Here's how the part is built. I have some questions about the finished solid (model axes, mm). A direction names the side the tool comes from. Round coordinates to 2 decimals unless told otherwise and drop trailing zeros. Order: outer loops, then holes, each group sorted by start corner. A loop starts at its lowest first (then second) coordinate and runs counter-clockwise, first axis right, second up. Notation, with made-up numbers: (-24, 11.25) - (1, 11.25) arc R23 ccw to (1, 19.25) - close; hole circle Ø1 at (69.5, 74.5). An arc over 180 degrees is marked (long way). One line per item, written item: value.
from build123d import *

# Parameters (mm, degrees)
BOSS_EXTRUDE1_DEPTH = 5
BOSS_EXTRUDE2_DEPTH = 32
CUT_EXTRUDE2_DEPTH  = 5
CUT_EXTRUDE3_DEPTH  = 5
SKETCH7_R           = 6.75
SKETCH7_R_2         = 1.75
C_L_NG_C_DEPTH      = 146.27301883
SKETCH8_W           = 40
SKETCH8_H           = 10
BOSS_EXTRUDE3_DEPTH = 55
CUT_EXTRUDE5_DEPTH  = 179.966477308
SKETCH10_R          = 1.75
SKETCH10_R_2        = 2.25
C_L_DEPTH           = 121.768719069
BOSS_EXTRUDE4_REACH = 179.37
CUT_EXTRUDE7_DEPTH  = 5
SKETCH14_R          = 4
CUT_EXTRUDE8_DEPTH  = 2.5
CUT_EXTRUDE9_START  = -2.5
SKETCH15_R          = 4
CUT_EXTRUDE9_DEPTH  = 2.5
SKETCH16_W          = 6
SKETCH16_H          = 10.5
CUT_EXTRUDE10_DEPTH = 5
SKETCH20_W          = 110
SKETCH20_H          = 50.06
CUT_EXTRUDE11_DEPTH = 55
SKETCH22_R          = 2
CUT_EXTRUDE12_DEPTH = 5
CUT_EXTRUDE13_DEPTH = 1.5
CUT_EXTRUDE15_DEPTH = 89
SKETCH26_R          = 1.5
CUT_EXTRUDE16_DEPTH = 5


with BuildPart() as part:
    # Sketch1 → Boss-Extrude1 (new body)
    with BuildSketch(Plane(origin=(0, 0, 0), x_dir=(1, 0, 0), z_dir=(0, 1, 0))):
        Polygon((-25, 75), (-25, 42.5), (-70, 42.5), (-70, -42.5), (-25, -42.5), (-25, -75), (77, -75), (77, 75), align=None)
    extrude(amount=BOSS_EXTRUDE1_DEPTH)

    # Sketch3 → Boss-Extrude2 (add)
    with BuildSketch(Plane(origin=(0, 5, 0), x_dir=(1, 0, 0), z_dir=(0, 1, 0))):
        Polygon((-70, 25), (-65, 25), (-65, 37.5), (-17, 37.5), (-17, 27.5), (-12, 27.5), (-12, 42.5), (-70, 42.5), align=None)
        Polygon((-70, -25), (-70, -42.5), (-12, -42.5), (-12, -27.5), (-17, -27.5), (-17, -37.5), (-65, -37.5), (-65, -25), align=None)
    extrude(amount=BOSS_EXTRUDE2_DEPTH)

    # Sketch5 → Cut-Extrude2 (cut)
    with BuildSketch(Plane.ZY.offset(70)):
        Polygon((-25, 37), (-35, 37), (-35, 27), (-25, 5), align=None)
        Polygon((25, 5), (25, 37), (35, 37), (35, 27), align=None)
    extrude(amount=-CUT_EXTRUDE2_DEPTH, mode=Mode.SUBTRACT)

    # Sketch6 → Cut-Extrude3 (cut)
    with BuildSketch(Plane(origin=(-12, 0, 0), x_dir=(0, 0, -1), z_dir=(1, 0, 0))):
        Polygon((-27.5, 37), (-37.5, 37), (-37.5, 12), (-27.5, 5), align=None)
        Polygon((37.5, 12), (27.5, 5), (27.5, 37), (37.5, 37), align=None)
    extrude(amount=-CUT_EXTRUDE3_DEPTH, mode=Mode.SUBTRACT)

    # Sketch7 → c l_ _ng c (cut, through all)
    with BuildSketch(Plane(origin=(0, 0, -42.5), x_dir=(-1, 0, 0), z_dir=(0, 0, -1))):
        with Locations((49, 21)):
            Circle(SKETCH7_R)
        with Locations((25, 30)):
            Circle(SKETCH7_R_2)
        with Locations((25, 12)):
            Circle(SKETCH7_R_2)
        with Locations((58, 30)):
            Circle(SKETCH7_R_2)
        with Locations((58, 12)):
            Circle(SKETCH7_R_2)
    extrude(amount=-C_L_NG_C_DEPTH, mode=Mode.SUBTRACT)

    # Sketch8 → Boss-Extrude3 (add)
    with BuildSketch(Plane(origin=(0, 5, 0), x_dir=(1, 0, 0), z_dir=(0, 1, 0))):
        with Locations((57, -70)):
            Rectangle(SKETCH8_W, SKETCH8_H)
        with Locations((57, 70)):
            Rectangle(SKETCH8_W, SKETCH8_H)
    extrude(amount=BOSS_EXTRUDE3_DEPTH)

    # Sketch9 → Cut-Extrude5 (cut, through all)
    with BuildSketch(Plane(origin=(0, 0, -75), x_dir=(-1, 0, 0), z_dir=(0, 0, -1))):
        Polygon((-77, 0), (-37, 55.055276819), (-37, 60), (-77, 60), align=None)
    extrude(amount=-CUT_EXTRUDE5_DEPTH, mode=Mode.SUBTRACT)

    # Sketch10 → c L (cut, through all)
    with BuildSketch(Plane(origin=(0, 0, 0), x_dir=(-1, 0, 0), z_dir=(0, -1, 0))):
        with Locations(Location((-29, -12, 0), (0, 0, 90))):
            Circle(SKETCH10_R)
        with Locations(Location((-17, -46, 0), (0, 0, 90))):
            Circle(SKETCH10_R)
        with Locations(Location((-17, 46, 0), (0, 0, 90))):
            Circle(SKETCH10_R)
        with Locations(Location((-29, 12, 0), (0, 0, 90))):
            Circle(SKETCH10_R)
        with Locations(Location((-28, -69.5, 0), (0, 0, 90))):
            Circle(SKETCH10_R_2)
        with Locations(Location((8, -69.5, 0), (0, 0, 90))):
            Circle(SKETCH10_R_2)
        with Locations(Location((8, 69.5, 0), (0, 0, 90))):
            Circle(SKETCH10_R_2)
        with Locations(Location((-28, 69.5, 0), (0, 0, 90))):
            Circle(SKETCH10_R_2)
    extrude(amount=-C_L_DEPTH, mode=Mode.SUBTRACT)

    # Sketch11 → Boss-Extrude4 (add, up to next)
    with BuildSketch(Plane(origin=(0, 0, -75), x_dir=(-1, 0, 0), z_dir=(0, 0, -1)), mode=Mode.PRIVATE) as boss_extrude4_sk1:
        Polygon((-37, 55.055276819), (-37, 50.055276819), (-73.36728736, 0), (-77, 0), align=None)
    boss_extrude4_tool1 = extrude(boss_extrude4_sk1.sketch, amount=-BOSS_EXTRUDE4_REACH, mode=Mode.PRIVATE) - part.part
    add(boss_extrude4_tool1.solids().sort_by_distance((56.106222, 26.297459, -75))[0])

    # Sketch13 → Cut-Extrude7 (cut)
    with BuildSketch(Plane(origin=(50.397154283, 36.615675877, 0), x_dir=(0, 0, -1), z_dir=(0.8090169943749486, 0.5877852522924716, 0))):
        Polygon((-7.731971797, -31.499332186), (-52.405674619, -31.039898345), (-48.866988089, -10.026742728), (-4.277711394, -9.567044368), align=None)
        Polygon((53.010105385, -31.499464427), (49.555844988, -9.567176647), (3.94811969, -10.026742728), (7.33, -31.499464427), align=None)
    extrude(amount=-CUT_EXTRUDE7_DEPTH, mode=Mode.SUBTRACT)

    # Sketch14 → Cut-Extrude8 (cut)
    with BuildSketch(Plane(origin=(0, 0, 37.5), x_dir=(-1, 0, 0), z_dir=(0, 0, -1))):
        with Locations((58, 30)):
            Circle(SKETCH14_R)
        with Locations((25, 30)):
            Circle(SKETCH14_R)
        with Locations((25, 12)):
            Circle(SKETCH14_R)
        with Locations((58, 12)):
            Circle(SKETCH14_R)
        with BuildLine():
            Line((38.8, 26.25), (38.8, 15.75))
            ThreePointArc((38.8, 15.75), (36, 12.95), (33.2, 15.75))
            Line((33.2, 15.75), (33.2, 26.25))
            ThreePointArc((33.2, 26.25), (36, 29.05), (38.8, 26.25))
        make_face()
    extrude(amount=-CUT_EXTRUDE8_DEPTH, mode=Mode.SUBTRACT)

    # Sketch15 → Cut-Extrude9 (cut)
    with BuildSketch(Plane.XY.offset(-37.5).offset(CUT_EXTRUDE9_START)):
        with Locations(Location((-25, 30, 0), (0, 0, 180))):
            Circle(SKETCH15_R)
        with Locations(Location((-25, 12, 0), (0, 0, 180))):
            Circle(SKETCH15_R)
        with Locations(Location((-58, 12, 0), (0, 0, 180))):
            Circle(SKETCH15_R)
        with Locations(Location((-58, 30, 0), (0, 0, 180))):
            Circle(SKETCH15_R)
        with BuildLine():
            Line((-33.2, 26.25), (-33.2, 15.75))
            ThreePointArc((-33.2, 15.75), (-36, 12.95), (-38.8, 15.75))
            Line((-38.8, 15.75), (-38.8, 26.25))
            ThreePointArc((-38.8, 26.25), (-36, 29.05), (-33.2, 26.25))
        make_face()
    extrude(amount=CUT_EXTRUDE9_DEPTH, mode=Mode.SUBTRACT)

    # Sketch16 → Cut-Extrude10 (cut)
    with BuildSketch(Plane(origin=(0, 0, 0), x_dir=(-1, 0, 0), z_dir=(0, -1, 0))):
        with Locations((57, 0)):
            Rectangle(SKETCH16_W, SKETCH16_H)
        with Locations((-64, 0)):
            Rectangle(SKETCH16_W, SKETCH16_H)
    extrude(amount=-CUT_EXTRUDE10_DEPTH, mode=Mode.SUBTRACT)

    # Sketch20 → Cut-Extrude11 (cut)
    with BuildSketch(Plane.ZY.offset(-77)):
        with Locations((0, 30.025276819)):
            Rectangle(SKETCH20_W, SKETCH20_H)
    extrude(amount=CUT_EXTRUDE11_DEPTH, mode=Mode.SUBTRACT)

    # Sketch22 → Cut-Extrude12 (cut)
    with BuildSketch(Plane(origin=(50.397154283, 36.615675877, 0), x_dir=(0, 0, -1), z_dir=(0.8090169943749486, 0.5877852522924716, 0))):
        with Locations(Location((-61, 12.792600242, 0), (0, 0, 90))):
            Circle(SKETCH22_R)
        with Locations(Location((-61, -30.259464427, 0), (0, 0, 90))):
            Circle(SKETCH22_R)
        with Locations(Location((61, -30.259464427, 0), (0, 0, 270))):
            Circle(SKETCH22_R)
        with Locations(Location((61, 12.792600242, 0), (0, 0, 270))):
            Circle(SKETCH22_R)
    extrude(amount=-CUT_EXTRUDE12_DEPTH, mode=Mode.SUBTRACT)

    # Sketch23 → Cut-Extrude13 (cut)
    with BuildSketch(Plane(origin=(0, 5, 0), x_dir=(1, 0, 0), z_dir=(0, 1, 0))):
        Polygon((-7, 38.5), (-6, 38.5), (0, 38.5), (24.5, 38.5), (24.5, 53), (-7, 53), align=None)
        Polygon((24.5, -38.5), (24.5, -53), (-7, -53), (-7, -38.5), (-6, -38.5), (0, -38.5), align=None)
    extrude(amount=-CUT_EXTRUDE13_DEPTH, mode=Mode.SUBTRACT)

    # Sketch25 → Cut-Extrude15 (cut)
    with BuildSketch(Plane.XY.offset(42.5)):
        with BuildLine():
            Line((-70, 10.452488445), (-70, 0))
            Line((-70, 0), (-59.547511555, 0))
            ThreePointArc((-59.547511555, 0), (-65.617009358, 4.382990642), (-70, 10.452488445))
        make_face()
    extrude(amount=-CUT_EXTRUDE15_DEPTH, mode=Mode.SUBTRACT)

    # Sketch26 → Cut-Extrude16 (cut)
    with BuildSketch(Plane.XZ):
        with Locations(Location((-57.011914478, 11.55, 0), (0, 0, 270))):
            Circle(SKETCH26_R)
        with Locations(Location((-57.011914478, -11.55, 0), (0, 0, 90))):
            Circle(SKETCH26_R)
        with Locations(Location((-20, -55, 0), (0, 0, 270))):
            Circle(SKETCH26_R)
        with Locations(Location((-20, 55, 0), (0, 0, 90))):
            Circle(SKETCH26_R)
    extrude(amount=-CUT_EXTRUDE16_DEPTH, mode=Mode.SUBTRACT)


solid = part.part
Q1. If we section it at D-D, the plane x = -36: Please give me the cut outline in (y, z), then the cut area to 4 significant figures.
Results list:
outline: (0, -42.5) - (37, -42.5) - (37, -37.5) - (29.05, -37.5) - (29.05, -40) - (12.95, -40) - (12.95, -37.5) - (5, -37.5) - (5, 37.5) - (12.95, 37.5) - (12.95, 40) - (29.05, 40) - (29.05, 37.5) - (37, 37.5) - (37, 42.5) - (0, 42.5) - close
area: 664.5 mm²
Q2. If we section it at C-C, the plane y = 21: Give the number of separate pieces and of enclosed holes in the cut face, then the cut area to 3 significant figures.
Results list:
separate pieces: 6
enclosed holes: 0
area: 1,040 mm²
Q3. Will these pins go through, and if not, where does the flat tip stop? pin 1 (4 mm diameter, centred on x = -35, y = 25.5, fed in from +Z); pin 2 (9.5 mm diameter, centred on x = -42.5, y = 20.5, fed in from -Z); pin 3 (1.5 mm diameter, centred on x = 32.5, z = -35.5, fed in from +Y); pin 4 (3 mm diameter, centred on x = -5.5, z = 48.5, fed in from -Y).
Results list:
pin 1: z = 42.5
pin 2: z = -42.5
pin 3: y = 5
pin 4: y = 0
Q4. If we section it at B-B, the plane x = -15: Please give me the cut outline in (y, z).
Results list:
outline: (0, -75) - (5, -75) - (5, -42.5) - (37, -42.5) - (37, -37.5) - (12, -37.5) - (5, -27.5) - (5, 27.5) - (12, 37.5) - (37, 37.5) - (37, 42.5) - (5, 42.5) - (5, 75) - (0, 75) - close
Q5. We'd pull the mould along Z, two halves only. Please class faces 4 (the flat face through (41, 15, 75)), 5 (the flat face through (67, 2, 0)): released by +Z, released by -Z, zero draft, split by the parting line, or undercut.
Results list:
face 4: released by +Z
face 5: undercut
Q6. Which directions (+Z, -Z, +X, -X, +Y, -Y) give clear straight access to the entire face, cutting with the end or side of a thin tool? Please do faces 1 (the flat face through (-32, 21, 37.5)), 2 (the flat face through (-14.46, 8.55, 32.57)), 3 (the flat face through (-27, 31, -40)).
Results list:
face 1: +Y
face 2: +X, +Y
face 3: none
Q7. If I drill on line 1 along Y through (x, z) = (-58, 38); line 2 along Y through (x, z) = (-25, -41); line 3 along X through (y, z) = (1, 69), over which ranges is the centre line in solid material (lowest first)?
Results list:
line 1: 0 to 8, 16 to 26, 34 to 37
line 2: 0 to 10.25, 13.75 to 28.25, 31.75 to 37
line 3: -25 to -10.19, -5.81 to 25.81, 30.19 to 76.27
Q8. If we section it at A-A, the plane z = -46: Please give me the cut outline in (x, y).
Results list:
outline: (-25, 0) - (15.25, 0) - (15.25, 3.5) - (-7, 3.5) - (-7, 5) - (-25, 5) - close; (18.75, 0) - (77, 0) - (73.37, 5) - (24.5, 5) - (24.5, 3.5) - (18.75, 3.5) - close
